Verification items for the finished model (mm, model axes). A direction names the side the tool comes from. Round coordinates to 2 decimals unless told otherwise and drop trailing zeros. Order: outer loops, then holes, each group sorted by start corner. A loop starts at its lowest first (then second) coordinate and runs counter-clockwise, first axis right, second up. Notation, with made-up numbers: (-2, 44) -> (3, 44) arc R4 cw to (3, 51) -> close; hole circle Ø8 at (77, -10.75). An arc over 180 degrees is marked (long way). Return JSON: item names as keys, results as strings. Group by question number.
1) Section check D-D on z = -7.5. Enter the section's corners in (x, y), plus the area to 3 significant figures.
2) Depth check by flat-ended pin: pin 1 (1.3 mm diameter, centred on x = 0, y = 17.5, fed in from -Z); pin 2 (6 mm diameter, centred on x = -0.5, y = -1, fed in from +Z); pin 3 (6.5 mm diameter, centred on x = -1, y = 17.5, fed in from -Z); pin 4 (5 mm diameter, centred on x = -5.5, z = 2, fed in from -Y). Enter the tip coordinate at first touch or a pass-through.
3) Draft check along Y on faces 6 (the cylindrical face through (-9.8, -3.3, -5.6)), 7 (the cylindrical face through (0.1, 20.5, -8.5)), 8 (the cylindrical face through (-0.1, -20.5, -8.5)), 9 (the cylindrical face through (-9.78, -7.51, 4.39)). Enter one of: pulls with the +Y half, pulls with the -Y half, needs draft (parallel to the pull), parting line crosses it, or undercut.
4) Section check B-B on y = 0. Enter the section's corners in (x, z).
5) Section check C-C on z = 7.5. Enter the section's corners in (x, y).
6) Tool access check on faces 1 (the flat face through (-3, 15, -9)), 2 (the flat face through (-1, 12, 0)), 3 (the cylindrical face through (-9.776, 3.216, -5.649)), 4 (the flat face through (0, 16, -10)), 5 (the cylindrical face through (-0.698, 0.253, -11.497)). Record the directions out of +Z, -Z, +X, -X, +Y, -Y that give a thin tool (end or side, any length) a straight path to the whole face; none if there is none.
7) Section check A-A on x = 0. Enter the section's corners in (y, z), plus the area to 3 significant figures.
8) Scan lines: L1, parallel to X at y = 17.5, z = -9.3; L2, parallel to X at y = -6, z = 13; L3, parallel to Y at x = -9, z = -11. Record each from-to range of solid material in increasing order.
```python
from build123d import *

# Parameters (mm, degrees)
SKETCH_1_W          = 23
SKETCH_1_H          = 25
EXTRUDE_1_DEPTH     = 15
SKETCH_2_W          = 19.6
SKETCH_2_H          = 11.5
SKETCH_4_W          = 3.4
SKETCH_4_H          = 25
EXTRUDE_2_DEPTH     = 15
SKETCH_6_R          = 1.2
SKETCH_6_R_2        = 6.5
CUT_EXTRUDE_1_DEPTH = 4
SKETCH_8_R          = 1.1
EXTRUDE_3_DEPTH     = 8
SKETCH_8_2_R        = 1.1
CUT_EXTRUDE_4_DEPTH = 5
SKETCH_7_W          = 35
SKETCH_7_H          = 40
CUT_EXTRUDE_3_DEPTH = 5
FILLET_1_R          = 1


with BuildPart() as part:
    # Sketch 1 → Extrude 1 (new body)
    with BuildSketch(Plane.XY):
        Rectangle(SKETCH_1_W, SKETCH_1_H)
    extrude(amount=-EXTRUDE_1_DEPTH)

    # Sketch 2 → Cut-Revolve 2 (revolve, cut)
    with BuildSketch(Plane.XY):
        with Locations((1.7, -5.75)):
            Rectangle(SKETCH_2_W, SKETCH_2_H)
    revolve(axis=Axis((11.5, 0, 0), (-1, 0, 0)), mode=Mode.SUBTRACT)

    # Sketch 4 → Extrude 2 (add)
    with BuildSketch(Plane.XY):
        with Locations((-9.8, 0)):
            Rectangle(SKETCH_4_W, SKETCH_4_H)
    extrude(amount=EXTRUDE_2_DEPTH)

    # Sketch 6 → Cut-Extrude 1 (cut)
    with BuildSketch(Plane(origin=(-8.1, 0, 0), x_dir=(0, 0, -1), z_dir=(1, 0, 0))):
        with Locations((7.5, 0)):
            Circle(SKETCH_6_R)
        with Locations((3.75, -6.495190528)):
            Circle(SKETCH_6_R)
        with Locations((-3.75, -6.495190528)):
            Circle(SKETCH_6_R)
        Circle(SKETCH_6_R_2)
        with Locations((-7.5, 0)):
            Circle(SKETCH_6_R)
        with Locations((-3.75, 6.495190528)):
            Circle(SKETCH_6_R)
        with Locations((3.75, 6.495190528)):
            Circle(SKETCH_6_R)
    extrude(amount=-CUT_EXTRUDE_1_DEPTH, mode=Mode.SUBTRACT)

    # Sketch 8 → Extrude 3 (add)
    # profile 1 of 2: a face of its own
    with BuildSketch(Plane(origin=(0, 0, -15), x_dir=(-1, 0, 0), z_dir=(0, 0, -1))):
        with BuildLine():
            Line((3, 17.5), (3, 12.5))
            Line((3, 12.5), (-3, 12.5))
            Line((-3, 12.5), (-3, 17.5))
            ThreePointArc((-3, 17.5), (0, 20.5), (3, 17.5))
        make_face()
        with Locations(Location((0, 17.5, 0), (0, 0, 180))):
            Circle(SKETCH_8_R, mode=Mode.SUBTRACT)
    # profile 2 of 2: a face of its own
    with BuildSketch(Plane(origin=(0, 0, -15), x_dir=(-1, 0, 0), z_dir=(0, 0, -1))):
        with BuildLine():
            Line((-3, -17.5), (-3, -12.5))
            Line((-3, -12.5), (3, -12.5))
            Line((3, -12.5), (3, -17.5))
            ThreePointArc((3, -17.5), (0, -20.5), (-3, -17.5))
        make_face()
        with Locations((0, -17.5)):
            Circle(SKETCH_8_R, mode=Mode.SUBTRACT)
    extrude(amount=-EXTRUDE_3_DEPTH)

    # Sketch 8_2 → Cut-Extrude 4 (cut)
    # profile 1 of 2: a face of its own
    with BuildSketch(Plane(origin=(0, 0, -15), x_dir=(-1, 0, 0), z_dir=(0, 0, -1))):
        with BuildLine():
            Line((3, 17.5), (3, 12.5))
            Line((3, 12.5), (-3, 12.5))
            Line((-3, 12.5), (-3, 17.5))
            ThreePointArc((-3, 17.5), (0, 20.5), (3, 17.5))
        make_face()
        with Locations(Location((0, 17.5, 0), (0, 0, 180))):
            Circle(SKETCH_8_2_R, mode=Mode.SUBTRACT)
    # profile 2 of 2: a face of its own
    with BuildSketch(Plane(origin=(0, 0, -15), x_dir=(-1, 0, 0), z_dir=(0, 0, -1))):
        with BuildLine():
            Line((-3, -17.5), (-3, -12.5))
            Line((-3, -12.5), (3, -12.5))
            Line((3, -12.5), (3, -17.5))
            ThreePointArc((3, -17.5), (0, -20.5), (-3, -17.5))
        make_face()
        with Locations((0, -17.5)):
            Circle(SKETCH_8_2_R, mode=Mode.SUBTRACT)
    extrude(amount=-CUT_EXTRUDE_4_DEPTH, mode=Mode.SUBTRACT)

    # Sketch 7 → Cut-Extrude 3 (cut)
    with BuildSketch(Plane(origin=(11.5, 0, 0), x_dir=(0, 0, -1), z_dir=(1, 0, 0))):
        with Locations((11.5, 0)):
            Rectangle(SKETCH_7_W, SKETCH_7_H)
    extrude(amount=-CUT_EXTRUDE_3_DEPTH, mode=Mode.SUBTRACT)

    # Fillet 1
    fillet_1_edges = [part.edges().sort_by_distance(p)[0] for p in [
        (-2.5, 12.5, -15),
        (-11.5, 0, -15),
        (6.5, 0, -15),
        (-2.5, -12.5, -15),
    ]]
    fillet(fillet_1_edges, radius=FILLET_1_R)


solid = part.part
```
Check result:
{
 "1": {"outline": "(-11.5, -12.5) -> (-3, -12.5) -> (-3, -17.5) arc R3 ccw to (3, -17.5) -> (3, -12.5) -> (6.5, -12.5) -> (6.5, -8.72) -> (-8.1, -8.72) -> (-8.1, -1.2) -> (-11.5, -1.2) -> close; (-11.5, 1.2) -> (-8.1, 1.2) -> (-8.1, 8.72) -> (6.5, 8.72) -> (6.5, 12.5) -> (3, 12.5) -> (3, 17.5) arc R3 ccw to (-3, 17.5) -> (-3, 12.5) -> (-11.5, 12.5) -> close; hole circle Ø2.2 at (0, -17.5); hole circle Ø2.2 at (0, 17.5)", "area": "268 mm^2"},
 "2": {"pin 1": "through", "pin 2": "z = -10.78", "pin 3": "z = -10", "pin 4": "y = -12.5"},
 "3": {"face 6": "undercut", "face 7": "pulls with the +Y half", "face 8": "pulls with the -Y half", "face 9": "undercut"},
 "4": {"outline": "(-11.5, -14) arc R1 ccw to (-10.5, -15) -> (5.5, -15) arc R1 ccw to (6.5, -14) -> (6.5, -11.5) -> (-8.1, -11.5) -> (-8.1, -8.7) -> (-11.5, -8.7) -> close; (-11.5, 8.7) -> (-8.1, 8.7) -> (-8.1, 15) -> (-11.5, 15) -> close"},
 "5": {"outline": "(-11.5, -12.5) -> (-8.1, -12.5) -> (-8.1, -1.2) -> (-11.5, -1.2) -> close; (-11.5, 1.2) -> (-8.1, 1.2) -> (-8.1, 12.5) -> (-11.5, 12.5) -> close"},
 "6": {"face 1": "+Z, -Z, -X, +Y", "face 2": "+Z, +X, +Y, -Y", "face 3": "+X, -X", "face 4": "-Z, +X, -X, +Y", "face 5": "+Z, +X"},
 "7": {"outline": "(-20.5, -10) -> (-18.6, -10) -> (-18.6, -7) -> (-20.5, -7) -> close; (-16.4, -10) -> (-12.5, -10) -> (-12.5, -14) arc R1 ccw to (-11.5, -15) -> (11.5, -15) arc R1 ccw to (12.5, -14) -> (12.5, -10) -> (16.4, -10) -> (16.4, -7) -> (12.5, -7) -> (12.5, 0) -> (11.5, 0) arc R11.5 cw to (-11.5, 0) -> (-12.5, 0) -> (-12.5, -7) -> (-16.4, -7) -> close; (18.6, -10) -> (20.5, -10) -> (20.5, -7) -> (18.6, -7) -> close", "area": "202 mm^2"},
 "8": {"L1": "-3 to -1.1, 1.1 to 3", "L2": "-11.5 to -8.1", "L3": "-12.5 to 12.5"}
}
